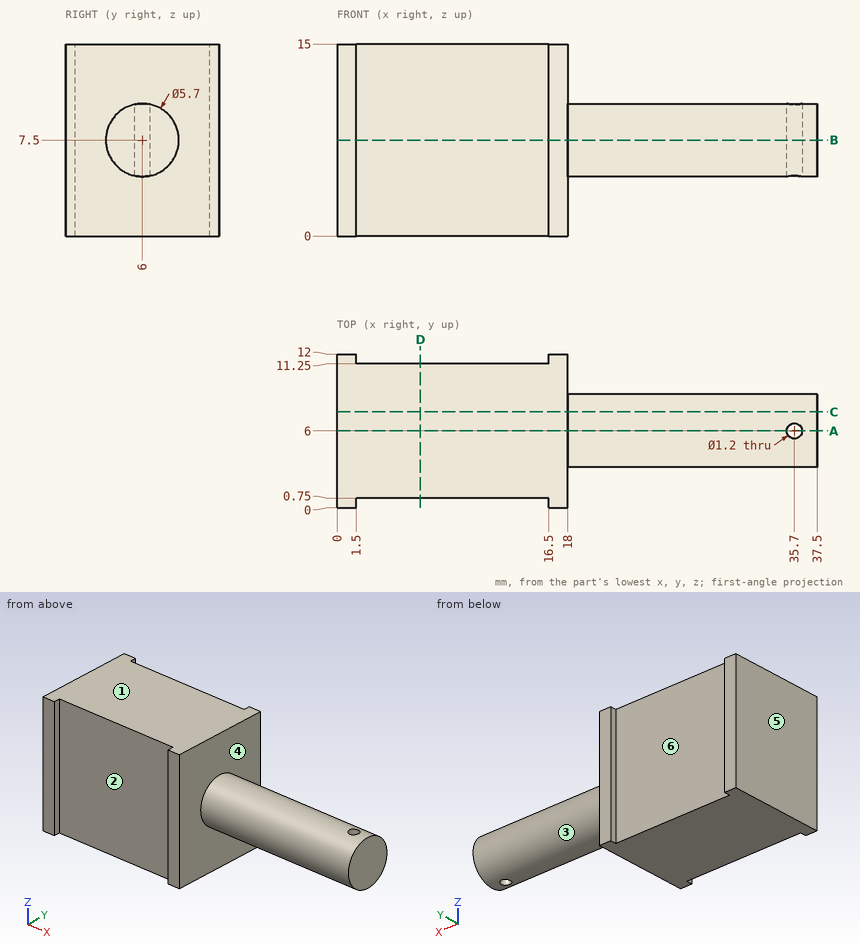
Input: dimensioned drawing with shaded views. Units: mm. Origin: part minimum x, y, z. A direction names the side the tool comes from. Round coordinates to 2 decimals unless told otherwise and drop trailing zeros. Order: outer loops, then holes, each group sorted by start corner. A loop starts at its lowest first (then second) coordinate and runs counter-clockwise, first axis right, second up. Notation, with made-up numbers: (64, 16.25) -> (115, 16.25) arc R15 ccw to (115, 24.25) -> close; hole circle Ø5 at (29, -33). An arc over 180 degrees is marked (long way). Put each result on its own line as item: value. Start each with the question number.
Q1. First-contact query: pin 1 (0.8 mm diameter, centred on y = 0.5, z = 8.5, fed in from +X); pin 2 (2 mm diameter, centred on x = 28, z = 2.5, fed in from -Y); pin 3 (1.4 mm diameter, centred on x = 35.7, y = 6, fed in from +Z); pin 4 (7.5 mm diameter, centred on x = 6, z = 5.5, fed in from -Y). Flat tips, straight axial feed; report the tip coordinate or a pass-through.
Q2. Section C-C on y = 7.5. Return the cut outline in (x, z).
Q3. Reachability of the marked faces 1, 2 and 3 from +Z, -Z, +X, -X, +Y, -Y: full face, straight path, thin tool, end or side. Return the list, or none.
Q4. Section B-B on z = 7.5. Return the cut outline in (x, y).
Q5. Section A-A on y = 6. Return the cut outline in (x, z).
Q6. Line query: probe 1 along Y at (x, z) = (3, 8.75); probe 2 along X at (y, z) = (1.75, 1); probe 3 along Y at (x, z) = (35.7, 6.9). Output: solid intervals per line, ascending.
Q7. Section D-D on x = 6.5. Return the cut outline in (y, z).
Q8. Pull-direction query (X, two-part tool) for the marked faces 4, 5 and 6; classes: +X half, -X half, draft (parallel to the pull), parting line (faces both ways), or undercut.
Ans:
1. pin 1: stops at x = 18
1. pin 2: passes through
1. pin 3: stops at z = 10.35
1. pin 4: stops at y = 0.75
2. outline: (0, 0) -> (18, 0) -> (18, 5.08) -> (37.5, 5.08) -> (37.5, 9.92) -> (18, 9.92) -> (18, 15) -> (0, 15) -> close
3. face 1: +Z, +X, -X, +Y, -Y
3. face 2: +Z, -Z, -Y
3. face 3: +X
4. outline: (0, 0) -> (1.5, 0) -> (1.5, 0.75) -> (16.5, 0.75) -> (16.5, 0) -> (18, 0) -> (18, 3.15) -> (37.5, 3.15) -> (37.5, 8.85) -> (18, 8.85) -> (18, 12) -> (16.5, 12) -> (16.5, 11.25) -> (1.5, 11.25) -> (1.5, 12) -> (0, 12) -> close; hole circle Ø1.2 at (35.7, 6)
5. outline: (0, 0) -> (18, 0) -> (18, 4.65) -> (35.1, 4.65) -> (35.1, 10.35) -> (18, 10.35) -> (18, 15) -> (0, 15) -> close; (36.3, 4.65) -> (37.5, 4.65) -> (37.5, 10.35) -> (36.3, 10.35) -> close
6. probe 1: y = 0.75 to 11.25
6. probe 2: x = 0 to 18
6. probe 3: y = 3.21 to 5.4, 6.6 to 8.79
7. outline: (0.75, 0) -> (11.25, 0) -> (11.25, 15) -> (0.75, 15) -> close
8. face 4: +X half
8. face 5: -X half
8. face 6: undercut
